```python
from build123d import *

# Parameters (mm, degrees)
F0_W     = 60
F0_H     = 120
F1_DEPTH = 20
F2_T     = -3
F3_W     = 10
F3_H     = 5
F4_DEPTH = 60
F5_DEPTH = 60


with BuildPart() as f1:
    # F0 (on Top) → F1 (new body)
    with BuildSketch(Plane.XY):
        Rectangle(F0_W, F0_H)
    extrude(amount=F1_DEPTH)

    # F2
    f2_openings = [f1.faces().sort_by_distance(p)[0] for p in [
        (0, 0, 20),
    ]]
    offset(amount=F2_T, openings=f2_openings)

    # F3 (on Front) → F4 (join)
    with BuildSketch(Plane.XZ):
        with Locations((0, 17.5)):
            Rectangle(F3_W, F3_H)
    extrude(amount=F4_DEPTH)

    # F3 (on Front) → F5 (join)
    with BuildSketch(Plane.XZ):
        with Locations((0, 17.5)):
            Rectangle(F3_W, F3_H)
    extrude(amount=-F5_DEPTH)


solid = f1.part
```
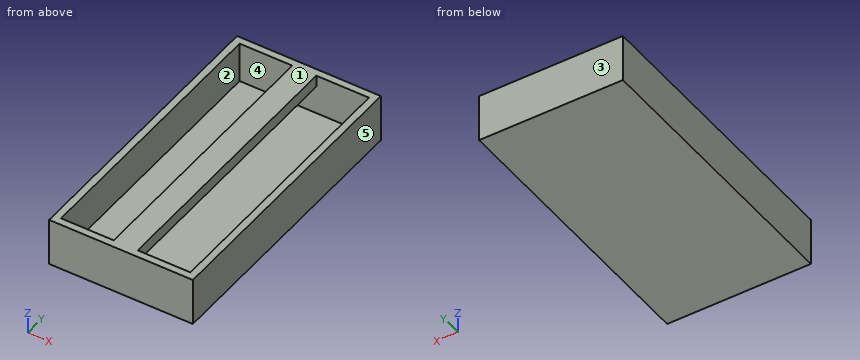
Geometry: final body of the model. Coordinates: model frame, mm. Face numbers are marked on the shaded views. A direction names the side the tool comes from. Round coordinates to 2 decimals unless told otherwise and drop trailing zeros. Order: outer loops, then holes, each group sorted by start corner. A loop starts at its lowest first (then second) coordinate and runs counter-clockwise, first axis right, second up. Notation, with made-up numbers: (-10, -14) -> (5, -14) arc R7 cw to (5, -1) -> close; hole circle Ø7 at (55.5, 75.25). An arc over 180 degrees is marked (long way). Use one line per item in the form item = value.
(1) First-contact query: pin 1 Ø4 at (x, y) = (6, 38.5) entering from +Z; pin 2 Ø8 at (x, y) = (-14, -34.5) entering from +Z. Flat tips, straight axial feed; report the tip coordinate or a pass-through.
Results list:
pin_1 = 20
pin_2 = 3
(2) Draft query along Y for the marked faces 3, 4 and 5. Return one class per face: pulls with the +Y half, pulls with the -Y half, needs draft (parallel to the pull), parting line crosses it, or undercut.
Results list:
face_3 = pulls with the +Y half
face_4 = undercut
face_5 = needs draft
(3) Section C-C on x = -23. Return loops of the section in (y, z).
Results list:
outline = (-60, 0) -> (60, 0) -> (60, 20) -> (57, 20) -> (57, 3) -> (-57, 3) -> (-57, 20) -> (-60, 20) -> close
(4) Section B-B on z = 16.25. Return loops of the section in (x, y), and give its area (3 significant figures).
Results list:
outline = (-30, -60) -> (30, -60) -> (30, 60) -> (-30, 60) -> close; hole (-27, -57) -> (-5, -57) -> (-5, 57) -> (-27, 57) -> close; hole (5, -57) -> (27, -57) -> (27, 57) -> (5, 57) -> close
area = 2,180 mm^2
(5) Access query for the marked faces 1 and 2. Directions: +Z, -Z, +X, -X, +Y, -Y. A direction counts if a zero-diameter tool reaches every point of the face in a straight line with its end or side. Return the directions, or none.
Results list:
face_1 = +Z, +X, -X, +Y, -Y
face_2 = +Z
(6) Section D-D on x = 0. Return loops of the section in (y, z).
Results list:
outline = (-60, 0) -> (60, 0) -> (60, 20) -> (-60, 20) -> close; hole (-57, 3) -> (57, 3) -> (57, 15) -> (-57, 15) -> close
(7) Ray query, probe 1 along Y at (x, z) = (20.5, 15.25); probe 2 along X at (y, z) = (40.5, 10.5); probe 3 along Z at (x, y) = (2, 32.5). Return the intervals inside material, ascending. Write a range as [from, to].
Results list:
probe_1 = [-60, -57], [57, 60]
probe_2 = [-30, -27], [27, 30]
probe_3 = [0, 3], [15, 20]
(8) Section A-A on y = -41.5. Return loops of the section in (x, z).
Results list:
outline = (-30, 0) -> (30, 0) -> (30, 20) -> (27, 20) -> (27, 3) -> (-27, 3) -> (-27, 20) -> (-30, 20) -> close; (-5, 15) -> (5, 15) -> (5, 20) -> (-5, 20) -> close
